Can you work these out from the drawing? Everything is in mm from the part's minimum corner. Coordinates: 2 decimals unless noted, no trailing zeros. Order: outer loops, then holes, each group sorted by start corner. A loop starts at its lowest first (then second) coordinate and runs counter-clockwise, first axis right, second up. Notation, with made-up numbers: (17, 51.5) -> (36, 51.5) arc R28 cw to (36, 85.5) -> close; hole circle Ø10 at (-35.5, 89). An arc over 180 degrees is marked (long way). Put each result on its own line as item: value. Start each with the question number.
Q1. If we section it at B-B (x = 3): Please give me the cut outline in (y, z).
Q2. If we section it at A-A (y = 51.5): Please give me the cut outline in (x, z).
Q3. Please list where these lines run through material, in increasing order: line 1 along X through (y, z) = (44, 0.9); line 2 along X through (y, z) = (34.5, 0.3); line 3 along Y through (x, z) = (13.5, 2.3) (1 decimal).
Q4. If we section it at C-C (z = 0.5): Please give me the cut outline in (x, y), and give its area (3 significant figures).
Q5. Will these pins go through, and if not, where does the flat tip stop? pin 1 (1.5 mm diameter, centred on y = 17, z = 2.5, fed in from +X); pin 2 (5 mm diameter, centred on x = 23.5, y = 22, fed in from -Z); pin 3 (0.9 mm diameter, centred on y = 32.5, z = 2, fed in from -X); pin 4 (0.9 mm diameter, centred on x = 13, z = 1.5, fed in from +Y).
Q6. If we section it at D-D (x = 46.5): Please give me the cut outline in (y, z).
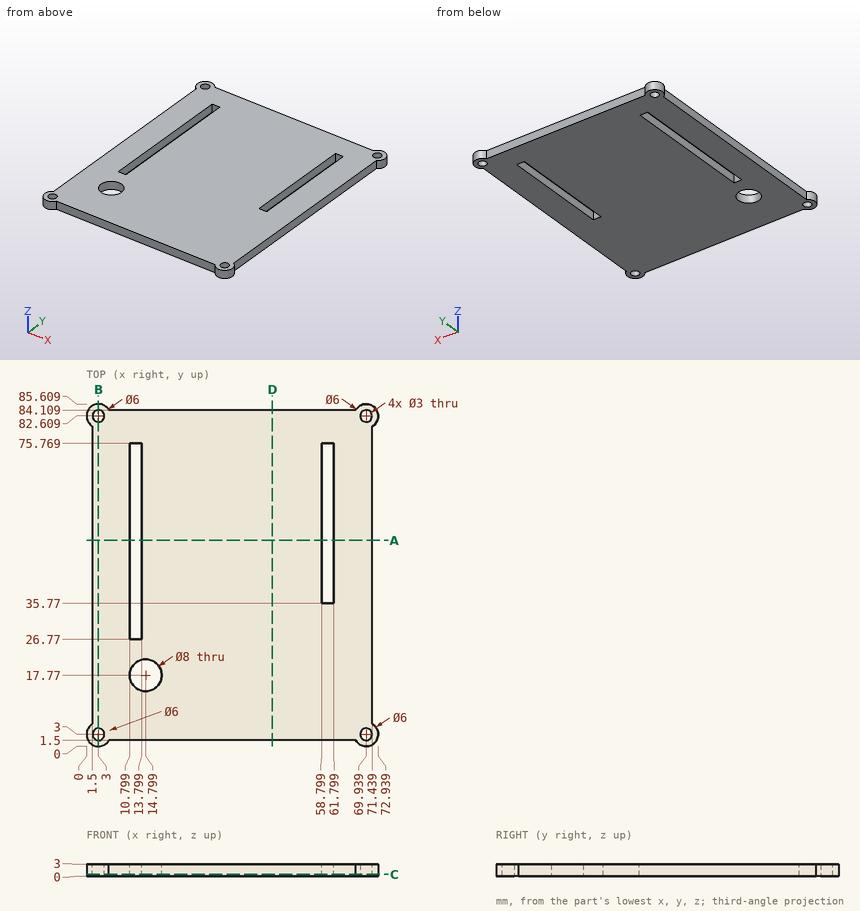
The answers:
1. outline: (0, 0) -> (1.5, 0) -> (1.5, 3) -> (0, 3) -> close; (4.5, 0) -> (81.11, 0) -> (81.11, 3) -> (4.5, 3) -> close; (84.11, 0) -> (85.61, 0) -> (85.61, 3) -> (84.11, 3) -> close
2. outline: (1.5, 0) -> (10.8, 0) -> (10.8, 3) -> (1.5, 3) -> close; (13.8, 0) -> (58.8, 0) -> (58.8, 3) -> (13.8, 3) -> close; (61.8, 0) -> (71.44, 0) -> (71.44, 3) -> (61.8, 3) -> close
3. line 1: 1.5 to 10.8, 13.8 to 58.8, 61.8 to 71.44
3. line 2: 1.5 to 10.8, 13.8 to 71.44
3. line 3: 1.5 to 14, 21.6 to 26.8, 75.8 to 84.1
4. outline: (1.5, 5.6) arc R3 ccw (long way) to (5.6, 1.5) -> (67.34, 1.5) arc R3 ccw (long way) to (71.44, 5.6) -> (71.44, 80.01) arc R3 ccw (long way) to (67.34, 84.11) -> (5.6, 84.11) arc R3 ccw (long way) to (1.5, 80.01) -> close; hole circle Ø3 at (3, 3); hole circle Ø3 at (3, 82.61); hole circle Ø8 at (14.8, 17.77); hole (10.8, 26.77) -> (13.8, 26.77) -> (13.8, 75.77) -> (10.8, 75.77) -> close; hole (58.8, 35.77) -> (61.8, 35.77) -> (61.8, 75.77) -> (58.8, 75.77) -> close; hole circle Ø3 at (69.94, 3); hole circle Ø3 at (69.94, 82.61)
4. area: 5,470 mm^2
5. pin 1: x = 71.44
5. pin 2: z = 0
5. pin 3: x = 1.5
5. pin 4: y = 84.11
6. outline: (1.5, 0) -> (84.11, 0) -> (84.11, 3) -> (1.5, 3) -> close
